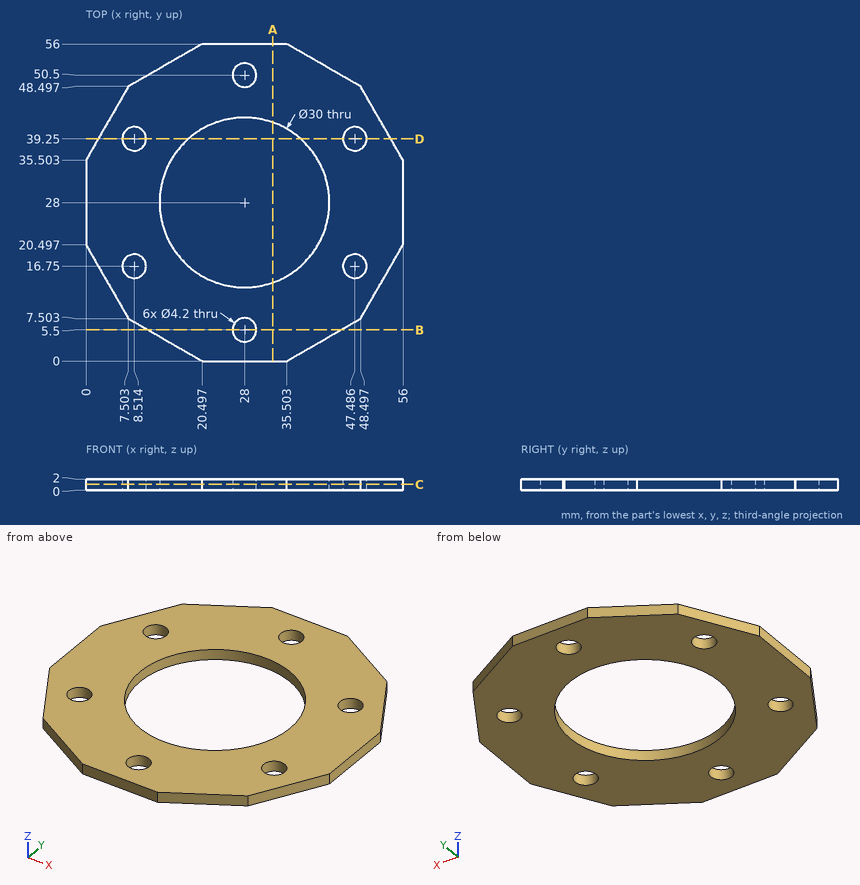
Geometry check sheet. Reference: drawing and pictorial views, mm from the part's lowest x, y, z. Coordinates: 2 decimals unless noted, no trailing zeros. Order: outer loops, then holes, each group sorted by start corner. A loop starts at its lowest first (then second) coordinate and runs counter-clockwise, first axis right, second up.
Item 1: Section check B-B, the plane y = 5.5. Enter the section's corners in (x, z).
Filled in:
outline: (10.97, 0) - (25.9, 0) - (25.9, 2) - (10.97, 2) - close; (30.1, 0) - (45.03, 0) - (45.03, 2) - (30.1, 2) - close
Item 2: Depth check by flat-ended pin: pin 1 (4 mm diameter, centred on x = 47.49, y = 16.75, fed in from +Z). Enter the tip coordinate at first touch or a pass-through.
Filled in:
pin 1: passes through
Item 3: Section check D-D, the plane y = 39.25. Enter the section's corners in (x, z) (1 decimal).
Filled in:
outline: (2.2, 0) - (6.4, 0) - (6.4, 2) - (2.2, 2) - close; (10.6, 0) - (18.1, 0) - (18.1, 2) - (10.6, 2) - close; (37.9, 0) - (45.4, 0) - (45.4, 2) - (37.9, 2) - close; (49.6, 0) - (53.8, 0) - (53.8, 2) - (49.6, 2) - close
Item 4: Material ranges on L1, parallel to Y at x = 28, z = 1.55; L2, parallel to X at y = 39, z = 0.15; L3, parallel to Y at x = 46, z = 1 (1 decimal), recorded low to high.
Filled in:
L1: y = 0 to 3.4, 7.6 to 13, 43 to 48.4, 52.6 to 56
L2: x = 2.02 to 6.43, 10.6 to 17.8, 38.2 to 45.4, 49.57 to 53.98
L3: y = 6.1 to 15.3, 18.2 to 37.8, 40.7 to 49.9
Item 5: Section check C-C, the plane z = 1.05. Give the number of separate pieces and of enclosed holes in the cut face, then the cut area to 3 significant figures.
Filled in:
separate pieces: 1
enclosed holes: 7
area: 1,730 mm2
Item 6: Section check A-A, the plane x = 33. Enter the section's corners in (y, z).
Filled in:
outline: (0, 0) - (13.86, 0) - (13.86, 2) - (0, 2) - close; (42.14, 0) - (56, 0) - (56, 2) - (42.14, 2) - close
